Geometry: final body of the model. Coordinates: model frame, mm. A direction names the side the tool comes from. Coordinates: 2 decimals unless noted, no trailing zeros. Order: outer loops, then holes, each group sorted by start corner. A loop starts at its lowest first (then second) coordinate and runs counter-clockwise, first axis right, second up. Notation, with made-up numbers: (-31, 12.5) - (7, 12.5) arc R30 cw to (7, 50.5) - close; hole circle Ø3 at (-26.75, 7). An arc over 180 degrees is marked (long way). Use a Markdown table: item, result. Add a question column.
```python
from build123d import *

# Parameters (mm, degrees)
BOSS_EXTRU_1_DEPTH        = 24
TROU_START                = 4
TROU_TARAUD_M61_OUTLINE_R = 2.5
TROU_TARAUD_M61_DEPTH     = 28
ESQUISSE2_W               = 89
ESQUISSE2_H               = 84
ENL_V_MAT_EXTRU_1_DEPTH   = 3
ESQUISSE3_R               = 10
ENL_V_MAT_EXTRU_2_DEPTH   = 185.024454914
ESQUISSE9_R               = 10
ENL_V_MAT_EXTRU_3_DEPTH   = 20
ESQUISSE10_R              = 5
ENL_V_MAT_EXTRU_4_DEPTH   = 184.913022939


# Read off the part's stored shape, not the designer's step: Trou taraudé M61
with BuildPart() as part:
    # Esquisse1 → Boss.-Extru.1 (new body)
    with BuildSketch(Plane.XY):
        Polygon((0, 0), (0, 10), (6, 16), (58, 16), (74, 32), (174, 32), (180, 26), (180, 0), align=None)
    boss_extru_1 = extrude(amount=BOSS_EXTRU_1_DEPTH)

    # Esquisse5 → Dégagement M11 (revolve, cut)
    with BuildSketch(Plane(origin=(162, 4, 24), x_dir=(0, -1, 0), z_dir=(1, 0, 0))):
        Polygon((0, 0), (0, 19.201721238), (2, 18), (2, 0), align=None)
    d_gagement_m11 = revolve(axis=Axis((162, 4, 30.35), (0, 0, -1)), mode=Mode.SUBTRACT)

    # Trou taraudé M61 outline → Trou taraudé M61 (cut)
    with BuildSketch(Plane(origin=(0, 0, 0), x_dir=(1, 0, 0), z_dir=(0, 1, 0)).offset(TROU_START)):
        with Locations((162, -12)):
            Circle(TROU_TARAUD_M61_OUTLINE_R)
    trou_taraud_m61 = extrude(amount=TROU_TARAUD_M61_DEPTH, mode=Mode.SUBTRACT)

    # Symétrie1: Boss.-Extru.1, Dégagement M11, Trou taraudé M61 across Top Plane
    add(boss_extru_1.mirror(Plane(origin=(0, 0, 0), x_dir=(1, 0, 0), z_dir=(0, 1, 0))))
    add(d_gagement_m11.mirror(Plane(origin=(0, 0, 0), x_dir=(1, 0, 0), z_dir=(0, 1, 0))), mode=Mode.SUBTRACT)
    add(trou_taraud_m61.mirror(Plane(origin=(0, 0, 0), x_dir=(1, 0, 0), z_dir=(0, 1, 0))), mode=Mode.SUBTRACT)

    # Esquisse2 → Enlèv. mat.-Extru.1 (cut)
    with BuildSketch(Plane.XY.offset(24)):
        with Locations((39.5, 0)):
            Rectangle(ESQUISSE2_W, ESQUISSE2_H)
    extrude(amount=-ENL_V_MAT_EXTRU_1_DEPTH, mode=Mode.SUBTRACT)

    # Esquisse3 → Enlèv. mat.-Extru.2 (cut, through all)
    with BuildSketch(Plane.XY.offset(21)):
        with Locations((16, 0)):
            Circle(ESQUISSE3_R)
    extrude(amount=-ENL_V_MAT_EXTRU_2_DEPTH, mode=Mode.SUBTRACT)

    # Esquisse9 → Enlèv. mat.-Extru.3 (cut)
    with BuildSketch(Plane(origin=(0, 0, 0), x_dir=(-1, 0, 0), z_dir=(0, 0, -1))):
        with Locations((-132, 0)):
            Circle(ESQUISSE9_R)
    extrude(amount=-ENL_V_MAT_EXTRU_3_DEPTH, mode=Mode.SUBTRACT)

    # Esquisse10 → Enlèv. mat.-Extru.4 (cut, through all)
    with BuildSketch(Plane(origin=(0, 0, 20), x_dir=(-1, 0, 0), z_dir=(0, 0, -1))):
        with Locations((-132, 0)):
            Circle(ESQUISSE10_R)
    extrude(amount=-ENL_V_MAT_EXTRU_4_DEPTH, mode=Mode.SUBTRACT)


solid = part.part
```
1) Section query D-D (z = 18.25). Return the cut outline in (x, y).
2) Section query A-A (z = 2.25). Return the cut outline in (x, y).
3) Access query for faces 1 (the cylindrical face through (162.766, 2.153, 15.126)), 2 (the flat face through (84, 0, 23)), 3 (the cylindrical face through (159.5, 17.8, 11.9)). Directions: +Z, -Z, +X, -X, +Y, -Y. A direction counts if a zero-diameter tool reaches every point of the face in a straight line with its end or side. Return the directions, or none.
4) Section query B-B (x = 132). Return the cut outline in (y, z).
5) Section query C-C (y = 21). Return the cut outline in (x, z).
6) Line query: line 1 (Y direction, x = 16, z = 5); line 2 (X direction, y = 3, z = 4.75); line 3 (Y direction, x = 162, z = 18.25). Output: solid intervals per line, ascending. Write a range as from..to.
7) Draft query along Z for faces 4 (the flat face through (130, 5, 20)), 5 (the cylindrical face through (162.766, -2.153, 15.126)), 6 (the cylindrical face through (159.5, -17.8, 11.9)), 7 (the conical face through (161.656, -4.045, 5.007)). Return one class per face: released by +Z, released by -Z, zero draft, split by the parting line, or undercut.
8) First-contact query: pin 1 (10.5 mm diameter, centred on x = 34, z = 11, fed in from +Y); pin 2 (12 mm diameter, centred on x = 132, y = 0, fed in from -Z); pin 3 (0.6 mm diameter, centred on x = 164, z = 12, fed in from +Y). Flat tips, straight axial feed; report the tip coordinate or a pass-through.
From the geometry:
| question | item | result |
|---|---|---|
| 1 | outline | (0, -10) - (6, -16) - (58, -16) - (74, -32) - (174, -32) - (180, -26) - (180, 26) - (174, 32) - (74, 32) - (58, 16) - (6, 16) - (0, 10) - close; hole circle Ø20 at (16, 0); hole circle Ø20 at (132, 0); hole circle Ø4 at (162, -4); hole circle Ø4 at (162, 4) |
| 2 | outline | (0, -10) - (6, -16) - (58, -16) - (74, -32) - (174, -32) - (180, -26) - (180, 26) - (174, 32) - (74, 32) - (58, 16) - (6, 16) - (0, 10) - close; hole circle Ø20 at (16, 0); hole circle Ø20 at (132, 0) |
| 3 | face 1 | +Z |
| 3 | face 2 | +Z, -X, +Y, -Y |
| 3 | face 3 | +Y |
| 4 | outline | (-32, 0) - (-10, 0) - (-10, 20) - (-5, 20) - (-5, 24) - (-32, 24) - close; (5, 20) - (10, 20) - (10, 0) - (32, 0) - (32, 24) - (5, 24) - close |
| 5 | outline | (63, 0) - (180, 0) - (180, 24) - (84, 24) - (84, 21) - (63, 21) - close; hole circle Ø5 at (162, 12) |
| 6 | line 1 | y = -16..-10, 10..16 |
| 6 | line 2 | x = 0..6.46, 25.54..122.46, 141.54..180 |
| 6 | line 3 | y = -32..-6, -2..2, 6..32 |
| 7 | face 4 | released by -Z |
| 7 | face 5 | zero draft |
| 7 | face 6 | undercut |
| 7 | face 7 | released by +Z |
| 8 | pin 1 | stops at y = 16 |
| 8 | pin 2 | stops at z = 20 |
| 8 | pin 3 | stops at y = 4 |
